Autodesk Fusion 360 part; units mm, degrees
sketch "Sketch1" plane through (0, 0, 0) normal (0, 0, 1) x (1, 0, 0)
  line L0 (12.5, -12) -> (-12.5, -12)
  line L1 (-12.5, -12) -> (-12.5, 12)
  line L2 (-12.5, 12) -> (12.5, 12)
  line L3 (12.5, 12) -> (12.5, -12)
  line L4 (12.5, -12) -> (-12.5, 12) construction
  line L5 (-12.5, -12) -> (12.5, 12) construction
  dimension "d1" = 25
  dimension "d2" = 24
extrude "Extrude1" add sketch "Sketch1" along normal blind 1
sketch "Sketch2" plane through (0, 0, 1) normal (0, 0, 1) x (-1, 0, 0)
  line L0 (-12.5, -12) -> (12.5, -12)
  line L1 (12.5, -12) -> (12.5, 12)
  line L2 (12.5, 12) -> (-12.5, 12)
  line L3 (-12.5, 12) -> (-12.5, -12)
  line L4 (5, 7) -> (-3, 7)
  line L5 (-3, 7) -> (-3, -1)
  line L6 (-3, -1) -> (5, -1)
  line L7 (5, -1) -> (5, 7)
  dimension "d5" = 8
  dimension "d6" = 8
  dimension "d7" = 7.5
  dimension "d8" = 5
extrude "Extrude2" add sketch "Sketch2" along normal blind 3 contours L4 L5 L6 L7
sketch "Sketch3" plane through (0, 0, 4) normal (0, 0, 1) x (-1, 0, 0)
  line L0 (5, -1) -> (5, 7)
  line L1 (5, 7) -> (-3, 7)
  line L2 (-3, 7) -> (-3, -1)
  line L3 (-3, -1) -> (5, -1)
  line L4 (-3, 3) -> (5, 3)
  line L5 (1, -1) -> (1, 7)
  circle A0 centre (1, 3) radius 3.5
  dimension "d11" = 7
extrude "Extrude3" add sketch "Sketch3" along normal blind 2 contours L4 L5 A0 | L4 L5 A0 | L4 L5 A0 | L4 L5 A0
fillet "Fillet1" radius 1 4 edges at (-12.5, -12, 0.5) (12.5, 12, 0.5) (12.5, -12, 0.5) (-12.5, 12, 0.5)
Check sheet for the modelled part. Datum: model origin and axes. Units: mm. A direction names the side the tool comes from. Round coordinates to 2 decimals unless told otherwise and drop trailing zeros. Write each loop counter-clockwise with the first axis right and the second up, starting at its lowest first coordinate (ties: lowest second). Pieces come first, ordered by that corner, then holes. Notation, with made-up numbers: (1, 55) - (44, 55) arc R35 ccw to (44, 94) - close; hole circle Ø10 at (11, 66.5). An arc over 180 degrees is marked (long way). Return JSON: item names as keys, results as strings.
Q1. Access from +Z, -Z, +X, -X, +Y, -Y to the whole of each face (thin tool, end or side, straight path). Record for faces 1 (the cylindrical face through (-0.241, -6.417, 4.986)), 2 (the flat face through (-1, 1, 2)), 3 (the flat face through (3, -3, 2)).
Returned:
{"face 1": "+Z", "face 2": "+Z, +X, -X, +Y", "face 3": "+Z, +X, +Y, -Y"}
Q2. Cross-section at A-A (x = -1). Record the boundary of the cut face in (y, z), then the cut area to 3 significant figures.
Returned:
{"outline": "(-12, 0) - (12, 0) - (12, 1) - (1, 1) - (1, 4) - (0.5, 4) - (0.5, 6) - (-6.5, 6) - (-6.5, 4) - (-7, 4) - (-7, 1) - (-12, 1) - close", "area": "62.0 mm²"}
Q3. Cross-section at B-B (y = -3). Record the boundary of the cut face in (x, z), then the cut area to 3 significant figures.
Returned:
{"outline": "(-12.5, 0) - (12.5, 0) - (12.5, 1) - (3, 1) - (3, 4) - (2.5, 4) - (2.5, 6) - (-4.5, 6) - (-4.5, 4) - (-5, 4) - (-5, 1) - (-12.5, 1) - close", "area": "63.0 mm²"}
Q4. Cross-section at D-D (y = 8.75). Record the boundary of the cut face in (x, z), then the cut area to 3 significant figures.
Returned:
{"outline": "(-12.5, 0) - (12.5, 0) - (12.5, 1) - (-12.5, 1) - close", "area": "25.0 mm²"}
Q5. Scan lines: L1, parallel to Z at x = 4.25, y = -5.5; L2, parallel to X at y = -1, z = 3.7; L3, parallel to Y at x = -3, z = 2.25. Record each from-to range of solid material in increasing order. Write a range as from..to.
Returned:
{"L1": "z = 0..1", "L2": "x = -5..3", "L3": "y = -7..1"}
Q6. Depth check by flat-ended pin: P1, Ø3, axis at x = -10, z = 3, coming from the +Y side; P2, Ø2.5, axis at x = -1, z = 2.5, coming from the -Y side; P3, Ø1.5, axis at x = -1, z = 2.5, coming from the +Y side; P4, Ø12, axis at x = 7.5, y = 3, coming from the +Z side. Enter the tip coordinate at first touch or a pass-through.
Returned:
{"P1": "passes through", "P2": "stops at y = -7", "P3": "stops at y = 1", "P4": "stops at z = 4"}
Q7. Cross-section at C-C (z = 1.65). Record the boundary of the cut face in (x, y).
Returned:
{"outline": "(-5, -7) - (3, -7) - (3, 1) - (-5, 1) - close"}
